Source: CAD feature listing. Evaluate the final solid. Frame: model axes, mm. Coordinates: 2 decimals unless noted, no trailing zeros. Order: outer loops, then holes, each group sorted by start corner. A loop starts at its lowest first (then second) coordinate and runs counter-clockwise, first axis right, second up.
Autodesk Inventor part; units mm, degrees
ref_plane "YZ Plane" through (0, 0, 0) normal (1, 0, 0) x (0, 1, 0)
ref_plane "XZ Plane" through (0, 0, 0) normal (0, 1, 0) x (-1, 0, 0)
ref_plane "XY Plane" through (0, 0, 0) normal (0, 0, 1) x (1, 0, 0)
sketch "Sketch1" plane through (0, 0, 0) normal (0, 0, 1) x (1, 0, 0)
  line L0 (0, 0) -> (15.24, 0)
  line L1 (15.24, 0) -> (15.24, -2.54)
  line L2 (15.24, -2.54) -> (0, -2.54)
  line L3 (0, -2.54) -> (0, 0)
  dimension "d0" = 15.24
  dimension "d1" = 2.54
extrude "Extrusion1" add sketch "Sketch1" along normal blind 2.54
sketch "Sketch2" plane through (0, 0, 2.54) normal (0, 0, 1) x (1, 0, 0)
  line L0 (15.24, 0) -> (0, 0)
  line L1 (0, 0) -> (0, -2.54)
  circle A0 centre (1.27, -1.27) radius 0.3175
  circle A1 centre (3.81, -1.27) radius 0.3175
  circle A2 centre (6.35, -1.27) radius 0.3175
  circle A3 centre (8.89, -1.27) radius 0.3175
  circle A4 centre (11.43, -1.27) radius 0.3175
  circle A5 centre (13.97, -1.27) radius 0.3175
  dimension "d4" = 0.635
  dimension "d6" = 1.27
  dimension "d9" = 2.54
extrude "Extrusion2" cut sketch "Sketch2" against normal blind 2.54
properties part number "Main Header" material "ABS Plastic"
Q1. Section query B-B on z = 1.9. Give the number of separate pieces and of enclosed holes in the cut face, plus the area to 3 significant figures.
Solutions:
separate pieces: 1
enclosed holes: 6
area: 36.8 mm2
Q2. Section query A-A on x = 13.97. Output: boundary loops of the cut face in (y, z).
Solutions:
outline: (-2.54, 0) - (-1.59, 0) - (-1.59, 2.54) - (-2.54, 2.54) - close; (-0.95, 0) - (0, 0) - (0, 2.54) - (-0.95, 2.54) - close
Q3. Material intervals for line 1 along Y through (x, z) = (14, 1.45); line 2 along Y through (x, z) = (13.75, 0.2), sorted ascending.
Solutions:
line 1: y = -2.54 to -1.59, -0.95 to 0
line 2: y = -2.54 to -1.5, -1.04 to 0
